Check sheet for the drawn part. Datum: minimum x, y, z corner. Units: mm. A direction names the side the tool comes from. Coordinates: 2 decimals unless noted, no trailing zeros. Order: outer loops, then holes, each group sorted by start corner. A loop starts at its lowest first (then second) coordinate and runs counter-clockwise, first axis right, second up.
1. Cross-section at D-D (x = 26). Enter the section's corners in (y, z), then the cut area to 3 significant figures.
2. Cross-section at A-A (x = 17). Enter the section's corners in (y, z).
3. Cross-section at C-C (z = 8.5). Enter the section's corners in (x, y), then the cut area to 3 significant figures.
4. Draft check along X on the marked faces 1, 2 and 3. Enter one of: released by +X, released by -X, zero draft, split by the parting line, or undercut.
5. Gauge pin test, flat ends, axial feed: pin 1 Ø4 at (x, y) = (26.5, 16) entering from -Z; pin 2 Ø10 at (x, y) = (28, 2.5) entering from +Z; pin 3 Ø5.5 at (x, z) = (17.5, 17.5) entering from -Y. Record the tip position at first contact, or that the pin passes through.
6. Cross-section at B-B (z = 16.5). Enter the section's corners in (x, y), then the cut area to 3 significant figures.
7. Thickness scan on line 1 (Y direction, x = 17, z = 29.5); line 2 (Z direction, x = 16.5, y = 3.25); line 3 (Z direction, x = 14, y = 1). Record the ranges inside material, lowest first.
8. Set-up check for the marked faces 4 and 5: record each of +Z, -Z, +X, -X, +Y, -Y from which the full face is reachable in a straight line by a thin tool's end or side.
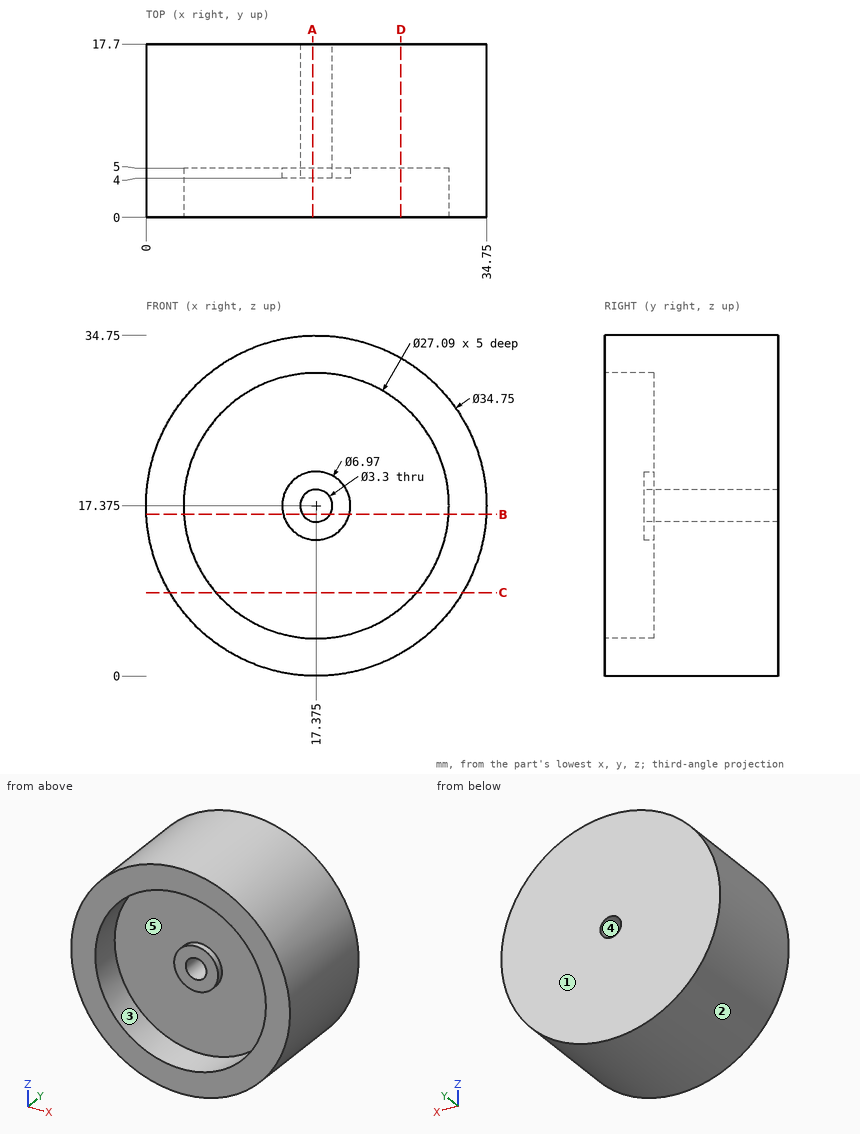
Data:
1. outline: (0, 2.29) - (17.7, 2.29) - (17.7, 32.46) - (0, 32.46) - (0, 27.82) - (5, 27.82) - (5, 6.93) - (0, 6.93) - close
1. area: 430 mm2
2. outline: (0, 0) - (17.7, 0) - (17.7, 15.77) - (4, 15.77) - (4, 13.91) - (5, 13.91) - (5, 3.84) - (0, 3.84) - close; (0, 30.91) - (5, 30.91) - (5, 20.84) - (4, 20.84) - (4, 18.98) - (17.7, 18.98) - (17.7, 34.75) - (0, 34.75) - close
3. outline: (2.44, 0) - (7.14, 0) - (7.14, 5) - (27.61, 5) - (27.61, 0) - (32.31, 0) - (32.31, 17.7) - (2.44, 17.7) - close
3. area: 426 mm2
4. face 1: zero draft
4. face 2: split by the parting line
4. face 3: undercut
5. pin 1: stops at z = 1.53
5. pin 2: stops at z = 33.81
5. pin 3: stops at y = 4
6. outline: (0.02, 0) - (3.86, 0) - (3.86, 5) - (14, 5) - (14, 4) - (15.98, 4) - (15.98, 17.7) - (0.02, 17.7) - close; (18.77, 4) - (20.75, 4) - (20.75, 5) - (30.89, 5) - (30.89, 0) - (34.73, 0) - (34.73, 17.7) - (18.77, 17.7) - close
6. area: 448 mm2
7. line 1: y = 5 to 17.7
7. line 2: z = 0.02 to 3.86, 30.89 to 34.73
7. line 3: z = 0.33 to 4.26, 30.49 to 34.42
8. face 4: +Y, -Y
8. face 5: -Y
